```python
from build123d import *

# Parameters (mm, degrees)
F1_W     = 87.5
F1_H     = 40
F1_W_2   = 8
F1_H_2   = 3
F1_R     = 1.5
F2_DEPTH = 3
F4_D     = 4.4
F5_R     = 5


with BuildPart() as f2:
    # F1 (on Top) → F2 (new body)
    with BuildSketch(Plane.XY):
        with Locations((-11.25, 0)):
            Rectangle(F1_W, F1_H)
        with Locations((-47, -14.4)):
            Rectangle(F1_W_2, F1_H_2, mode=Mode.SUBTRACT)
        with Locations((-39, -14.4)):
            Circle(F1_R, mode=Mode.SUBTRACT)
        with Locations((-24.5, -14)):
            Circle(F1_R, mode=Mode.SUBTRACT)
        with Locations((24.5, -14)):
            Circle(F1_R, mode=Mode.SUBTRACT)
        with Locations((-47, 14.4)):
            Rectangle(F1_W_2, F1_H_2, mode=Mode.SUBTRACT)
        with Locations((-39, 14.4)):
            Circle(F1_R, mode=Mode.SUBTRACT)
        with Locations((-24.5, 14)):
            Circle(F1_R, mode=Mode.SUBTRACT)
        with Locations((24.5, 14)):
            Circle(F1_R, mode=Mode.SUBTRACT)
    extrude(amount=F2_DEPTH)

    # F4 (through all)
    with Locations(Plane.XY.offset(3)):
        with Locations((-12.5, 6.125), (-12.5, -6.375), (12.5, 6.125), (12.5, -6.375)):
            Hole(F4_D / 2)

    # F5
    f5_edges = [f2.edges().sort_by_distance(p)[0] for p in [
        (32.5, 20, 1.5),
        (32.5, -20, 1.5),
    ]]
    fillet(f5_edges, radius=F5_R)


solid = f2.part
```
The model under review builds one solid part; all positions refer to its coordinate system, in mm. A direction names the side the tool comes from. Round coordinates to 2 decimals unless told otherwise and drop trailing zeros. Order: outer loops, then holes, each group sorted by start corner. A loop starts at its lowest first (then second) coordinate and runs counter-clockwise, first axis right, second up. Notation, with made-up numbers: M -21,-30 L 29,-30 A24 ccw 29,0 Z; hole C -26,40 d2. An arc over 180 degrees is marked long. Use a Markdown table: item, result.
1) Consider section C-C (x = 12.5). Write out the cut boundary in (y, z) (3 decimals).
Report:
| item | result |
|---|---|
| outline | M -20,0 L -8.575,0 L -8.575,3 L -20,3 Z; M -4.175,0 L 3.925,0 L 3.925,3 L -4.175,3 Z; M 8.325,0 L 20,0 L 20,3 L 8.325,3 Z |
2) Tool access review of faces 4 (the face through (-47, -15.9, 1)), 5 (the face through (-14, -20, 1)): name each direction out of +Z, -Z, +X, -X, +Y, -Y from which nothing blocks a thin tool from reaching the whole face with its end or side.
Report:
| item | result |
|---|---|
| face 4 | +Z, -Z |
| face 5 | +Z, -Z, +X, -X, -Y |
3) Draft analysis for pull direction X (two halves, no side actions). For faces 1 (the face through (32.5, 0, 1)), 2 (the face through (-55, 0, 1)), 3 (the face through (-43, 14, 1)), state which applies: released by +X, released by -X, zero draft, split by the parting line, or undercut.
Report:
| item | result |
|---|---|
| face 1 | released by +X |
| face 2 | released by -X |
| face 3 | undercut |
4) Insertion check: pin 1 (5.5 mm diameter, centred on x = -12.5, y = -6.375, fed in from -Z). The pin has a flat end and moves straight along its axis. Give the tip position at first contact, or say it passes through.
Report:
| item | result |
|---|---|
| pin 1 | z = 0 |
5) Consider section A-A (x = -39). Write out the cut boundary in (y, z), then the cut area to 3 significant figures.
Report:
| item | result |
|---|---|
| outline | M -20,0 L -15.9,0 L -15.9,3 L -20,3 Z; M -12.9,0 L 12.9,0 L 12.9,3 L -12.9,3 Z; M 15.9,0 L 20,0 L 20,3 L 15.9,3 Z |
| area | 102 mm^2 |
6) Wall thickness on line 1 along Y through (x, z) = (24.5, 2.4); line 2 along Y through (x, z) = (-47.5, 0.8); line 3 along X through (y, z) = (-7, 1.8): over which ranges is each line inside the solid? List them lowest first. Write a range as [from, to].
Report:
| item | result |
|---|---|
| line 1 | [-20, -15.5], [-12.5, 12.5], [15.5, 20] |
| line 2 | [-20, -15.9], [-12.9, 12.9], [15.9, 20] |
| line 3 | [-55, -14.61], [-10.39, 10.39], [14.61, 32.5] |
7) Consider section B-B (z = 1.4). Give the number of separate pieces and of enclosed holes in the cut face, then the cut area to 3 significant figures.
Report:
| item | result |
|---|---|
| separate pieces | 1 |
| enclosed holes | 12 |
| area | 3,340 mm^2 |
